Autodesk Inventor part; units mm, degrees
ref_plane "YZ Plane" through (0, 0, 0) normal (1, 0, 0) x (0, 1, 0)
ref_plane "XZ Plane" through (0, 0, 0) normal (0, 1, 0) x (-1, 0, 0)
ref_plane "XY Plane" through (0, 0, 0) normal (0, 0, 1) x (1, 0, 0)
sketch "Sketch1" plane through (0, 0, 0) normal (1, 0, 0) x (0, 1, 0)
  line L0 (0, 0) -> (0, -10.795)
  line L1 (0, -10.795) -> (2.54, -10.795)
  line L2 (0, 0) -> (12.7, 0)
  line L3 (2.54, -10.795) -> (2.54, -9.9414)
  line L4 (2.54, -9.9414) -> (2.54, -8.6714)
  line L5 (14.986, -3.937) -> (1.8235, -3.937) construction
  arc A0 (6.0461, -3.937) -> (2.54, -8.6714) centre (7.4896, -8.6714) ccw
  line L6 (9.398, -3.048) -> (9.398, -4.826)
  line L7 (6.0461, -3.937) -> (7.8921, -3.937)
  arc A1 (9.398, -4.826) -> (7.8921, -3.937) centre (7.8921, -5.6569) ccw
  line L8 (19.558, 0) -> (0, 0)
  line L9 (9.398, -3.048) -> (19.558, -3.048)
  line L10 (19.558, -3.048) -> (19.558, 0)
  dimension "d0" = 10.795
  dimension "d1" = 2.54
  dimension "d2" = 12.7
  dimension "d5" = 3.937
  dimension "d6" = 1.27
  dimension "d7" = 4.9496
  dimension "d18" = 4.826
  dimension "d19" = 1.7199
  dimension "d24" = 9.398
  dimension "d25" = 10.16
  dimension "d26" = 3.048
  dimension "d27" = 4.572
  dimension "d28" = 5.6234
  dimension "d29" = 17.7345
revolve "Revolution1" add sketch "Sketch1" angle 360 about axis through (0, 0, 0) along (0, 1, 0)
sketch "Sketch2" plane through (0, 0, 0) normal (0, -1, 0) x (1, 0, 0)
  circle A0 centre (0, 0) radius 3.048
  line L0 (4.95, -0.9536) -> (1.6491, -4.7636)
  line L1 (1.6491, -4.7636) -> (-3.3008, -3.81)
  line L2 (-3.3008, -3.81) -> (-4.95, 0.9536)
  line L3 (-4.95, 0.9536) -> (-1.6491, 4.7636)
  line L4 (-1.6491, 4.7636) -> (3.3008, 3.81)
  line L5 (3.3008, 3.81) -> (4.95, -0.9536)
  dimension "d11" = 8.7312
  dimension "d12" = 7.62
extrude "Extrusion1" cut sketch "Sketch2" against normal blind 3.302 contours A0 | L0 L1 L2 L3 L4 L5
sketch "Sketch3" plane through (0, 3.302, 0) normal (0, -1, 0) x (1, 0, 0)
  circle A0 centre (0, 0) radius 2.0892
  dimension "d15" = 4.1783
extrude "Extrusion2" cut sketch "Sketch3" against normal up to surface (16.256 mm away)
sketch "Sketch5" plane through (0, 9.398, 0) normal (0, 1, 0) x (1, 0, 0)
  circle A0 centre (0, 0) radius 4.826
  circle A1 centre (0, 0) radius 3.048
extrude "Extrusion5" add sketch "Sketch5" along normal blind 1.27
sketch "Sketch6" plane through (0, 0, 0) normal (0, -1, 0) x (1, 0, 0)
  circle A0 centre (0, 0) radius 3.048
  line L0 (-4.95, 0.9536) -> (-1.6491, 4.7636)
  circle A1 centre (0, 0) radius 5.041
extrude "Extrusion6" cut sketch "Sketch6" against normal up to surface (3.302 mm away)
sketch "Sketch7" plane through (0, 0, 0) normal (0, -1, 0) x (1, 0, 0)
  circle A0 centre (0, 0) radius 5.041
  circle A1 centre (0, 0) radius 10.795
extrude "Extrusion7" add sketch "Sketch7" along normal blind 1.016
fillet "Fillet1" radius 1.524 1 edges at (0, 2.54, 10.795)
properties part number "_3DPrint"
The model under review builds one solid part; all positions refer to its coordinate system, in mm. A direction names the side the tool comes from. Give positions to 0.01 mm unless a question says otherwise; leave off trailing zeros. Write each loop counter-clockwise with the first axis right and the second up, starting at its lowest first coordinate (ties: lowest second). Pieces come first, ordered by that corner, then holes. Notation, with made-up numbers: (-12, 33.5) -> (0, 33.5) arc R11 cw to (0, 41.5) -> close; hole circle Ø10 at (9, 23.5). An arc over 180 degrees is marked (long way). Answer in a Markdown table with one row per item.
1) For L1, parallel to Z at x = 0, y = 14.75; L2, parallel to X at y = 17.25, z = -1; L3, parallel to Y at x = -1.5, z = 8.5, list the stretches that pass through material, from the lowest coordinate up. Write a range as [from, to].
Worked answers:
| item | result |
|---|---|
| L1 | [-3.05, -2.09], [2.09, 3.05] |
| L2 | [-2.88, -1.83], [1.83, 2.88] |
| L3 | [-1.02, 2.54] |
2) Clearance check with flat-ended pins moving along their axes: P1, Ø3, axis at x = -1.5, z = -2, coming from the -Y side; P2, Ø3, axis at x = 3, z = 7.5, coming from the +Y side; P3, Ø3, axis at y = 13.5, z = -1.5, coming from the -X side. State where each tip first meets the part, or that it passes through.
Worked answers:
| item | result |
|---|---|
| P1 | y = 3.3 |
| P2 | y = 3 |
| P3 | x = -3.05 |
3) Mouldability with a two-part tool opening along Z and no side actions: class faces 4 (the flat face through (1, 10.668, 3.1)), 5 (the cylindrical face through (4.81, 1.11, 1.51)), 6 (the cylindrical face through (-3.83, 10.024, -2.937)) as +Z half, -Z half, draft (parallel to the pull), parting line (faces both ways), or undercut.
Worked answers:
| item | result |
|---|---|
| face 4 | draft |
| face 5 | undercut |
| face 6 | parting line |
4) Add section A-A on y = 17. State the section outline as (x, z) points.
Worked answers:
| item | result |
|---|---|
| outline | circle Ø6.1 at (0, 0); hole circle Ø4.18 at (0, 0) |
5) Tool access review of faces 1 (the flat face through (1, 3.302, -2.2)), 2 (the cylindrical face through (3.843, 6.982, 0.853)), 3 (the cylindrical face through (-3.02, 15.18, 0.4)): name each direction out of +Z, -Z, +X, -X, +Y, -Y from which nothing blocks a thin tool from reaching the whole face with its end or side.
Worked answers:
| item | result |
|---|---|
| face 1 | -Y |
| face 2 | none |
| face 3 | +Y |
6) Add section B-B on y = 5.25. State the section outline as (x, z) points, plus the area to 3 significant figures.
Worked answers:
| item | result |
|---|---|
| outline | circle Ø8.52 at (0, 0); hole circle Ø4.18 at (0, 0) |
| area | 43.2 mm² |
